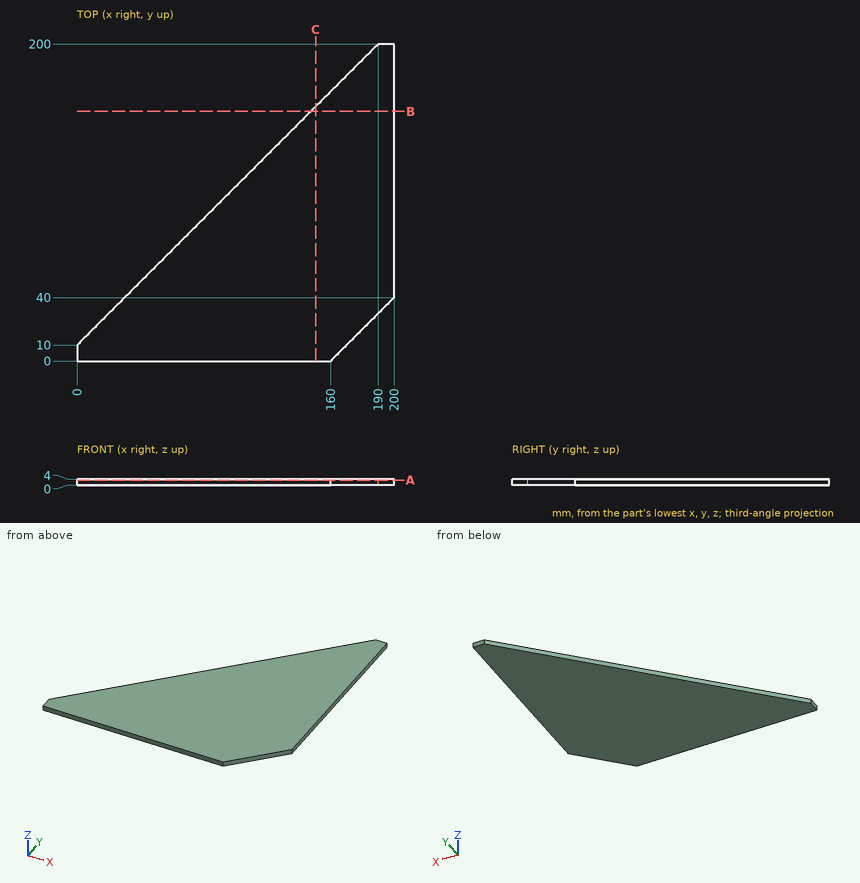
Job drawing, mm, ordinate dimensions from the low corner. One solid piece. Round coordinates to 2 decimals unless told otherwise and drop trailing zeros. Order: outer loops, then holes, each group sorted by start corner. A loop starts at its lowest first (then second) coordinate and runs counter-clockwise, first axis right, second up. Notation, with made-up numbers: (15, -11) -> (65, -11) arc R10 ccw to (65, 1) -> close; hole circle Ø2 at (5.25, 13). An arc over 180 degrees is marked (long way). Write item = value, one per line.
(1) Cut at C-C (x = 150.5). Write the cut outline in (y, z).
Answers follow:
outline = (0, 0) -> (160.5, 0) -> (160.5, 4) -> (0, 4) -> close
(2) Cut at A-A (z = 3.25). Write the cut outline in (x, y), plus the area to 4 significant figures.
Answers follow:
outline = (0, 0) -> (160, 0) -> (200, 40) -> (200, 200) -> (190, 200) -> (0, 10) -> close
area = 21,150 mm²
(3) Cut at B-B (y = 157.5). Write the cut outline in (x, z).
Answers follow:
outline = (147.5, 0) -> (200, 0) -> (200, 4) -> (147.5, 4) -> close
(4) Flat gauge pins, fed straight in: P1, Ø1, axis at y = 110.5, z = 1, coming from the -X side; P2, Ø1.5, axis at y = 42, z = 3.5, coming from the -X side. Where does each tip first touch, or does it go through?
Answers follow:
P1 = 100
P2 = 31.25
(5) Drill centre lines: L1, parallel to X at y = 18, z = 2.6; L2, parallel to X at y = 122, z = 2.8; L3, parallel to Y at x = 98.5, z = 1.6. Where is each one in solid material? Low to high.
Answers follow:
L1 = 8 to 178
L2 = 112 to 200
L3 = 0 to 108.5
